```python
from build123d import *

# Parameters (mm, degrees)
BOSS_EXTRUDE1_DEPTH = 3.175
SKETCH4_R           = 2.159
CUT_EXTRUDE2_DEPTH  = 216.549531721


with BuildPart() as part:
    # Sketch2 → Boss-Extrude1 (new body)
    with BuildSketch(Plane(origin=(0, 0, 0), x_dir=(1, 0, 0), z_dir=(0, 1, 0))):
        Polygon((-152.4, 116.478975516), (-116.478975516, 152.4), (116.478975516, 152.4), (152.4, 116.478975516), (152.4, -116.478975516), (116.478975516, -152.4), (-116.478975516, -152.4), (-152.4, -116.478975516), align=None)
        with BuildLine():
            Line((-116.478975516, 80.557951031), (-80.557951031, 116.478975516))
            Line((-80.557951031, 116.478975516), (-80.557951031, 120.65))
            ThreePointArc((-80.557951031, 120.65), (-76.838207153, 129.630256121), (-67.857951031, 133.35))
            Line((-67.857951031, 133.35), (67.857951031, 133.35))
            ThreePointArc((67.857951031, 133.35), (76.838207153, 129.630256121), (80.557951031, 120.65))
            Line((80.557951031, 120.65), (80.557951031, 116.478975516))
            Line((80.557951031, 116.478975516), (116.478975516, 80.557951031))
            Line((116.478975516, 80.557951031), (120.65, 80.557951031))
            ThreePointArc((120.65, 80.557951031), (129.630256121, 76.838207153), (133.35, 67.857951031))
            Line((133.35, 67.857951031), (133.35, -67.857951031))
            ThreePointArc((133.35, -67.857951031), (129.630256121, -76.838207153), (120.65, -80.557951031))
            Line((120.65, -80.557951031), (116.478975516, -80.557951031))
            Line((116.478975516, -80.557951031), (80.557951031, -116.478975516))
            Line((80.557951031, -116.478975516), (80.557951031, -120.65))
            ThreePointArc((80.557951031, -120.65), (76.838207153, -129.630256121), (67.857951031, -133.35))
            Line((67.857951031, -133.35), (-67.857951031, -133.35))
            ThreePointArc((-67.857951031, -133.35), (-76.838207153, -129.630256121), (-80.557951031, -120.65))
            Line((-80.557951031, -120.65), (-80.557951031, -116.478975516))
            Line((-80.557951031, -116.478975516), (-116.478975516, -80.557951031))
            Line((-116.478975516, -80.557951031), (-120.65, -80.557951031))
            ThreePointArc((-120.65, -80.557951031), (-129.630256121, -76.838207153), (-133.35, -67.857951031))
            Line((-133.35, -67.857951031), (-133.35, 67.857951031))
            ThreePointArc((-133.35, 67.857951031), (-129.630256121, 76.838207153), (-120.65, 80.557951031))
            Line((-120.65, 80.557951031), (-116.478975516, 80.557951031))
        make_face(mode=Mode.SUBTRACT)
    extrude(amount=BOSS_EXTRUDE1_DEPTH)

    # Sketch4 → Cut-Extrude2 (cut, through all)
    with BuildSketch(Plane(origin=(0, 3.175, 0), x_dir=(1, 0, 0), z_dir=(0, 1, 0))):
        with Locations(Location((0, 144.78, 0), (0, 0, 270))):
            Circle(SKETCH4_R)
        with Locations(Location((-50.8, 144.78, 0), (0, 0, 270))):
            Circle(SKETCH4_R)
        with Locations(Location((-144.78, 50.8, 0), (0, 0, 270))):
            Circle(SKETCH4_R)
        with Locations(Location((-144.78, 0, 0), (0, 0, 270))):
            Circle(SKETCH4_R)
        with Locations(Location((144.78, 0, 0), (0, 0, 90))):
            Circle(SKETCH4_R)
        with Locations(Location((144.78, 50.8, 0), (0, 0, 90))):
            Circle(SKETCH4_R)
        with Locations(Location((50.8, 144.78, 0), (0, 0, 90))):
            Circle(SKETCH4_R)
        with Locations(Location((50.8, -144.78, 0), (0, 0, 270))):
            Circle(SKETCH4_R)
        with Locations(Location((144.78, -50.8, 0), (0, 0, 270))):
            Circle(SKETCH4_R)
        with Locations(Location((-50.8, -144.78, 0), (0, 0, 90))):
            Circle(SKETCH4_R)
        with Locations(Location((0, -144.78, 0), (0, 0, 90))):
            Circle(SKETCH4_R)
        with Locations(Location((-144.78, -50.8, 0), (0, 0, 90))):
            Circle(SKETCH4_R)
    extrude(amount=-CUT_EXTRUDE2_DEPTH, mode=Mode.SUBTRACT)


solid = part.part
```
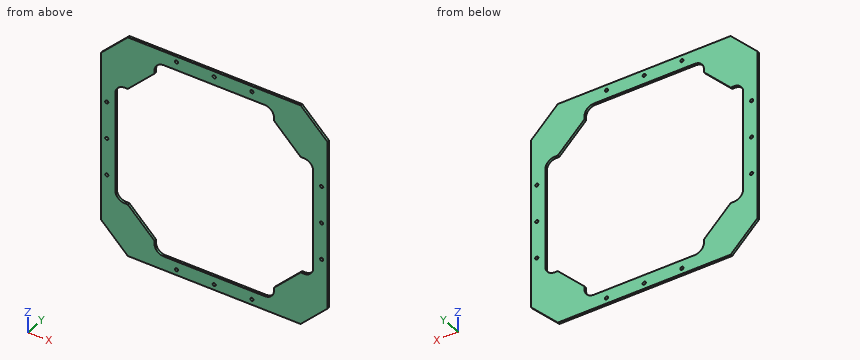
Check sheet for the modelled part. Datum: model origin and axes. Units: mm. Coordinates: 2 decimals unless noted, no trailing zeros. Loops run counter-clockwise (first coordinate to the right, second up) from the corner with the lowest first, then second, coordinate; pieces in that order, holes last.
1) Gauge pin test, flat ends, axial feed: pin 1 (1.6 mm diameter, centred on x = -119, y = 1.5, fed in from -Z); pin 2 (1 mm diameter, centred on y = 1, z = 119, fed in from +X); pin 3 (1 mm diameter, centred on y = 2, z = 119, fed in from -X). Record the tip position at first contact, or that the pin passes through.
2) Sectioned sample at B-B (z = 18). Record the boundary of the cut face in (x, y) (3 decimals).
3) Material ranges on probe 1 along X at (y, z) = (0.8, -50.8); probe 2 along X at (y, z) = (2, -41); probe 3 along Z at (x, y) = (-0.5, 1.7), recorded low to high.
4) Sectioned sample at A-A (x = 60). Record the boundary of the cut face in (y, z) (3 decimals), and give its area (3 significant figures).
5) Sectioned sample at C-C (y = 2.15). Count the separate pieces of the cut face and the enclosed holes in it, and give its area (3 significant figures).
Check sheet entries:
1. pin 1: stops at z = -150.68
1. pin 2: stops at x = 150.38
1. pin 3: stops at x = -150.38
2. outline: (-152.4, 0) - (-133.35, 0) - (-133.35, 3.175) - (-152.4, 3.175) - close; (133.35, 0) - (152.4, 0) - (152.4, 3.175) - (133.35, 3.175) - close
3. probe 1: x = -152.4 to -146.94, -142.62 to -133.35, 133.35 to 142.62, 146.94 to 152.4
3. probe 2: x = -152.4 to -133.35, 133.35 to 152.4
3. probe 3: z = -152.4 to -146.88, -142.68 to -133.35, 133.35 to 142.68, 146.88 to 152.4
4. outline: (0, -152.4) - (3.175, -152.4) - (3.175, -133.35) - (0, -133.35) - close; (0, 133.35) - (3.175, 133.35) - (3.175, 152.4) - (0, 152.4) - close
4. area: 121 mm2
5. separate pieces: 1
5. enclosed holes: 13
5. area: 27,900 mm2
